Answer from the drawing. Dimensions are ordinates in mm from the lowest x, y and z of the part. A direction names the side the tool comes from. Coordinates: 2 decimals unless noted, no trailing zeros. Write each loop counter-clockwise with the first axis right and the second up, starting at its lowest first coordinate (ties: lowest second). Pieces come first, ordered by that corner, then holes. Notation, with made-up numbers: (21, 40) -> (78, 40) arc R29 cw to (78, 62) -> close; hole circle Ø6 at (73.25, 85). An arc over 180 degrees is marked (long way). One line per item, written item: value. Start each with the question number.
1. Find section A-A, the plane z = 3. Write down the section's boundary in (x, y).
2. For a pull along Z with two mould halves and no side action, classify the marked faces 4, 5 and 6 as pulls with the +Z half, pulls with the -Z half, needs draft (parallel to the pull), parting line crosses it, or undercut.
3. Consider line 1 along X through (y, z) = (10, 2.05); line 2 along Z through (x, y) = (4.15, 2.75). Determine where each line is inside the solid, lowest interval first.
4. For the marked faces 1, 2 and 3, determine the directions among +Z, -Z, +X, -X, +Y, -Y from which every point of the face is accessible in a straight line to the end or side of a thin tool.
5. Given P1, Ø2, axis at y = 14, z = 1, coming from the +X side; P2, Ø1.5, axis at y = 11.5, z = 1.5, coming from the +X side; P3, Ø3, axis at x = 4.5, y = 10.5, coming from the +Z side; P4, Ø1.6, axis at x = 2.5, z = 2.5, coming from the -Y side, each flat-ended and moving along its own axis, determine where each tip first touches the part or whether it passes through.
6. Find section B-B, the plane y = 12.25. Write down the section's boundary in (x, z).
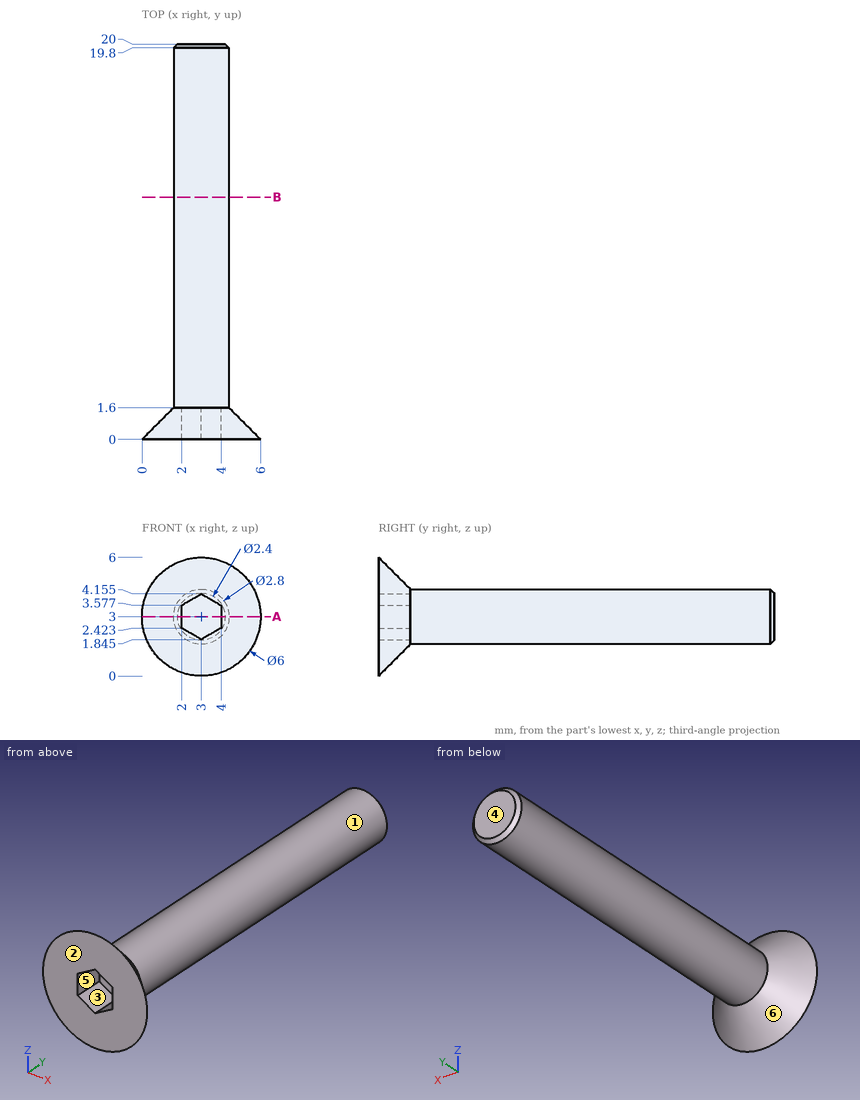
Answer block:
1. outline: (0, 0) -> (2, 0) -> (2, 1.6) -> (4, 1.6) -> (4, 0) -> (6, 0) -> (4.4, 1.6) -> (4.4, 19.8) -> (4.2, 20) -> (1.8, 20) -> (1.6, 19.8) -> (1.6, 1.6) -> close
2. face 4: needs draft
2. face 5: undercut
2. face 6: parting line crosses it
3. line 1: x = 1.97 to 4.03
3. line 2: z = 2.2 to 3.8
4. face 1: +Y
4. face 2: +Z, -Z, +X, -X, -Y
4. face 3: -Y
5. P1: stops at x = 3.98
5. P2: stops at x = 4.18
5. P3: stops at z = 4.4
5. P4: stops at y = 0
6. outline: circle Ø2.8 at (3, 3)
